```python
from build123d import *

# Parameters (mm, degrees)
SKIZZE1_R                       = 60
AUFSATZ_LINEAR_AUSTRAGEN1_DEPTH = 30
SKIZZE2_R                       = 20
AUFSATZ_LINEAR_AUSTRAGEN2_DEPTH = 360
SKIZZE3_R                       = 40
AUFSATZ_LINEAR_AUSTRAGEN3_DEPTH = 35
AUFSATZ_LINEAR_START            = 20
SKIZZE4_R                       = 60
AUFSATZ_LINEAR_AUSTRAGEN4_DEPTH = 20


with BuildPart() as part:
    # Skizze1 → Aufsatz-Linear austragen1 (new body)
    with BuildSketch(Plane.XY):
        Circle(SKIZZE1_R)
    extrude(amount=AUFSATZ_LINEAR_AUSTRAGEN1_DEPTH)

    # Skizze2 → Aufsatz-Linear austragen2 (add)
    with BuildSketch(Plane.XY.offset(30)):
        with Locations(Location((0, 0, 0), (0, 0, 180))):
            Circle(SKIZZE2_R)
    extrude(amount=AUFSATZ_LINEAR_AUSTRAGEN2_DEPTH)

    # Skizze3 → Aufsatz-Linear austragen3 (add)
    with BuildSketch(Plane(origin=(0, 0, 0), x_dir=(-1, 0, 0), z_dir=(0, 0, -1))):
        Circle(SKIZZE3_R)
    extrude(amount=AUFSATZ_LINEAR_AUSTRAGEN3_DEPTH)

    # Skizze4 → Aufsatz-Linear austragen4 (add)
    with BuildSketch(Plane(origin=(0, 0, -35), x_dir=(-1, 0, 0), z_dir=(0, 0, -1)).offset(AUFSATZ_LINEAR_START)):
        with Locations(Location((0, 0, 0), (0, 0, 180))):
            Circle(SKIZZE4_R)
    extrude(amount=-AUFSATZ_LINEAR_AUSTRAGEN4_DEPTH)


solid = part.part
```
Input: part model. Units: mm. Frame: model coordinates. A direction names the side the tool comes from. Coordinates: 2 decimals unless noted, no trailing zeros. Write each loop counter-clockwise with the first axis right and the second up, starting at its lowest first coordinate (ties: lowest second). Pieces come first, ordered by that corner, then holes.
1) Set-up query: faces 1 (the cylindrical face through (19.98, -0.88, 207.48)), 2 (the flat face through (12, -39, 0)), 3 (the flat face through (0, 0, 390)). Return all of +Z, -Z, +X, -X, +Y, -Y with unobstructed straight access to the full face (end or side cutting, diameter ignored); none if empty.
2) Material intervals for line 1 along Z through (x, y) = (22.5, -51); line 2 along Z through (x, y) = (-30.5, -7); line 3 along X through (y, z) = (-6.5, 41), sorted ascending.
3) Section B-B on y = 0. Output: boundary loops of the cut face in (x, z), and give its area (3 significant figures).
4) Pin query (flat end, axial travel): pin 1 Ø3 at (x, z) = (-12.5, 301.5) entering from +Y; pin 2 Ø3 at (x, z) = (0, 339.5) entering from -Y; pin 3 Ø8 at (x, z) = (-27, 274.5) entering from +Y. Return the tip coordinate at first contact, or that it passes through.
5) Section D-D on z = 236. Output: boundary loops of the cut face in (x, y).
6) Section A-A on x = -45. Output: boundary loops of the cut face in (y, z).
7) Mould query, pull axis Z, two halves, no side actions, for faces 4 (the flat face through (12, 39, -35)), 5 (the cylindrical face through (8.67, -39.05, -17.26)), 6 (the cylindrical face through (-59.94, 2.64, 14.79)), 7 (the flat face through (26, 1, 30)). Classes: pulls with the +Z half, pulls with the -Z half, needs draft (parallel to the pull), parting line crosses it, or undercut.
Check result:
1. face 1: +Z
1. face 2: none
1. face 3: +Z, +X, -X, +Y, -Y
2. line 1: z = -55 to -35, 0 to 30
2. line 2: z = -55 to 30
2. line 3: x = -18.91 to 18.91
3. outline: (-60, -55) - (60, -55) - (60, -35) - (40, -35) - (40, 0) - (60, 0) - (60, 30) - (20, 30) - (20, 390) - (-20, 390) - (-20, 30) - (-60, 30) - (-60, 0) - (-40, 0) - (-40, -35) - (-60, -35) - close
3. area: 23,200 mm2
4. pin 1: stops at y = 16.7
4. pin 2: stops at y = -20
4. pin 3: passes through
5. outline: circle Ø40 at (0, 0)
6. outline: (-39.69, -55) - (39.69, -55) - (39.69, -35) - (-39.69, -35) - close; (-39.69, 0) - (39.69, 0) - (39.69, 30) - (-39.69, 30) - close
7. face 4: undercut
7. face 5: undercut
7. face 6: needs draft
7. face 7: pulls with the +Z half
